Check sheet for the modelled part. Datum: model origin and axes. Units: mm. Coordinates: 2 decimals unless noted, no trailing zeros. Order: outer loops, then holes, each group sorted by start corner. A loop starts at its lowest first (then second) coordinate and runs counter-clockwise, first axis right, second up.
from build123d import *

# Parameters (mm, degrees)
CYLINDER1793_R         = 74
CYLINDER1793_DEPTH     = 60
BOX751_W               = 80
BOX751_H               = 6
BOX751_DEPTH           = 20
BOX751_PLACEMENT_ANGLE = 20
BOX753_W               = 57
BOX753_H               = 6
BOX753_DEPTH           = 32


with BuildPart() as obj1:
    # Cylinder1793 → Cylinder1793 (new body)
    with BuildSketch(Plane.XY.offset(26)):
        Circle(CYLINDER1793_R)
    extrude(amount=CYLINDER1793_DEPTH)


with BuildPart() as krychle751:
    # Box751 → Box751 (new body)
    with BuildSketch(Plane.XY):
        with Locations((40, 3)):
            Rectangle(BOX751_W, BOX751_H)
    extrude(amount=BOX751_DEPTH)


with BuildPart() as krychle751_1:
    # Box751 placement: moved
    add(krychle751.part.moved(Location((-131.7, -24, 54.35))).rotate(Axis((-131.7, -24, 54.35), (0, 1, 0)), BOX751_PLACEMENT_ANGLE))


with BuildPart() as cut554:
    # Box753 → Box753 (new body)
    with BuildSketch(Plane(origin=(-122, -24, 52), x_dir=(1, 0, 0), z_dir=(0, 0, 1))):
        with Locations((28.5, 3)):
            Rectangle(BOX753_W, BOX753_H)
    extrude(amount=BOX753_DEPTH)

    # Cut553: cut Krychle751
    add(krychle751_1.part, mode=Mode.SUBTRACT)

    # Cut554: cut obj1
    add(obj1.part, mode=Mode.SUBTRACT)


solid = cut554.part
(1) Cross-section at B-B (x = -83.5). Enter the section's corners in (y, z), and give its area (3 significant figures).
Filled in:
outline: (-24, 58.09) - (-18, 58.09) - (-18, 84) - (-24, 84) - close
area: 155 mm2
(2) Go/stop test with a flat-tipped pin: P1, Ø1, axis at x = -110.5, y = -22, coming from the -Z side. Record where the tip stops, or that it passes through.
Filled in:
P1: stops at z = 67.74
(3) Thickness scan on probe 1 along Z at (x, y) = (-76, -18.25); probe 2 along Z at (x, y) = (-84, -19.25); probe 3 along X at (y, z) = (-20.5, 76). Record the ranges inside material, lowest first.
Filled in:
probe 1: z = 55.36 to 84
probe 2: z = 58.27 to 84
probe 3: x = -122 to -71.1
(4) Cross-section at A-A (z = 80). Enter the section's corners in (x, y).
Filled in:
outline: (-122, -24) - (-70, -24) arc R74 cw to (-71.78, -18) - (-122, -18) - close
